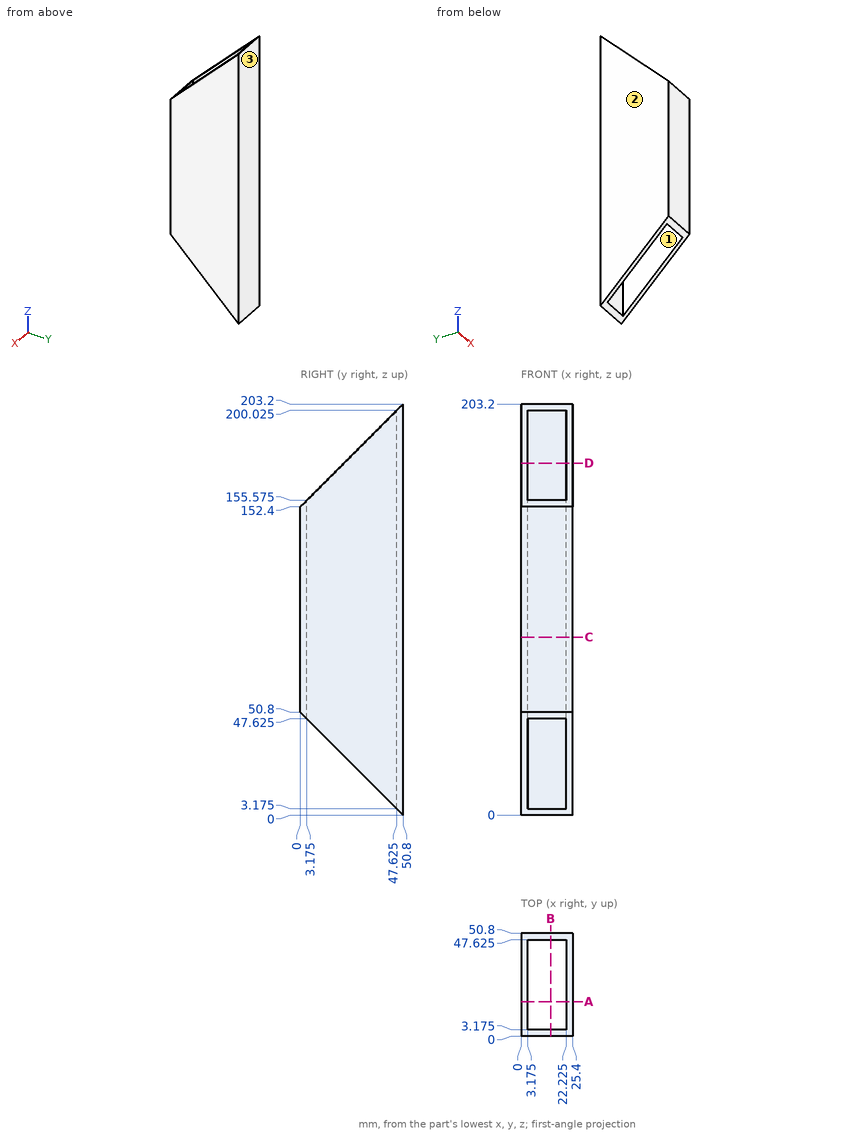
Design review of the part shown in the three views and the two pictorial views. Dimensions are in mm from the part's minimum x, y and z. Coordinates: 2 decimals unless noted, no trailing zeros. Order: outer loops, then holes, each group sorted by start corner. A loop starts at its lowest first (then second) coordinate and runs counter-clockwise, first axis right, second up.
1) Take a section at C-C, the plane z = 88. Give the boundary of the cut face in (x, y) (3 decimals), and give its area (3 significant figures).
2) Take a section at D-D, the plane z = 174. Give the boundary of the cut face in (x, y) (3 decimals).
3) Wall thickness on line 1 along X through (y, z) = (47.5, 127.5) (3 decimals); line 2 along Y through (x, z) = (7.75, 23.5) (3 decimals); line 3 along Y through (x, z) = (10.25, 78) (3 decimals): over which ranges is each line inside the solid? List them lowest first.
4) Take a section at A-A, the plane y = 17. Give the boundary of the cut face in (x, z) (3 decimals).
5) Take a section at B-B, the plane x = 14.5. Give the boundary of the cut face in (y, z) (3 decimals).
6) Mouldability with a two-part tool opening along Y and no side actions: class the marked faces 1, 2 and 3 as +Y half, -Y half, draft (parallel to the pull), parting line (faces both ways), or undercut.
7) Clearance check with flat-ended pins moving along their axes: pin 1 (6 mm diameter, centred on x = 3.5, y = 16, fed in from +Z); pin 2 (2 mm diameter, centred on x = 15, z = 164, fed in from -Y) (3 decimals); pin 3 (10 mm diameter, centred on x = 5.5, y = 25.5, fed in from +Z); pin 4 (5 mm diameter, centred on x = 19.5, y = 9, fed in from +Z). State where each tip first meets the part, or that it passes through.
Returned:
1. outline: (0, 0) - (25.4, 0) - (25.4, 50.8) - (0, 50.8) - close; hole (3.175, 3.175) - (22.225, 3.175) - (22.225, 47.625) - (3.175, 47.625) - close
1. area: 444 mm2
2. outline: (0, 21.6) - (3.175, 21.6) - (3.175, 47.625) - (22.225, 47.625) - (22.225, 21.6) - (25.4, 21.6) - (25.4, 50.8) - (0, 50.8) - close
3. line 1: x = 0 to 3.175, 22.225 to 25.4
3. line 2: y = 47.625 to 50.8
3. line 3: y = 0 to 3.175, 47.625 to 50.8
4. outline: (0, 33.8) - (3.175, 33.8) - (3.175, 169.4) - (0, 169.4) - close; (22.225, 33.8) - (25.4, 33.8) - (25.4, 169.4) - (22.225, 169.4) - close
5. outline: (0, 50.8) - (3.175, 47.625) - (3.175, 155.575) - (0, 152.4) - close; (47.625, 3.175) - (50.8, 0) - (50.8, 203.2) - (47.625, 200.025) - close
6. face 1: undercut
6. face 2: draft
6. face 3: +Y half
7. pin 1: stops at z = 171.38
7. pin 2: stops at y = 47.625
7. pin 3: stops at z = 182.33
7. pin 4: passes through
